Source: CAD feature listing. Evaluate the final solid. Frame: model axes, mm. A direction names the side the tool comes from. Coordinates: 2 decimals unless noted, no trailing zeros. Loops run counter-clockwise (first coordinate to the right, second up) from the corner with the lowest first, then second, coordinate; pieces in that order, holes last. Notation, with made-up numbers: (36.25, -22.5) -> (80.25, -22.5) arc R8 cw to (80.25, -11.5) -> close; hole circle Ø7 at (82.5, -18). An arc over 180 degrees is marked (long way). Answer as a JSON object with one key per item and string values. Group by question number.
from build123d import *

# Parameters (mm, degrees)
F0_W     = 450
F0_H     = 450
F1_DEPTH = 950
F2_W     = 50
F2_H     = 50
F2_H_2   = 425
F2_W_2   = 330
F3_DEPTH = 450.001
F4_W     = 380
F4_H     = 425
F5_DEPTH = 450.001
F6_W     = 380
F6_H     = 50
F6_H_2   = 306.2882968217
F7_DEPTH = 134.2592361444


with BuildPart() as f1:
    # F0 (on Top) → F1 (new body)
    with BuildSketch(Plane.XY):
        Rectangle(F0_W, F0_H)
    extrude(amount=F1_DEPTH)

    # F2 (on face) → F3 (cut, through all)
    with BuildSketch(Plane.YZ.offset(225)):
        Polygon((-225, 475), (140, 475), (190, 950), (-225, 950), align=None)
        Polygon((175, 475), (225, 475), (225, 950), align=None)
        with Locations((200, 450)):
            Rectangle(F2_W, F2_H)
        with Locations((200, 212.5)):
            Rectangle(F2_W, F2_H_2)
        with Locations((-25, 212.5)):
            Rectangle(F2_W_2, F2_H_2)
    extrude(amount=-F3_DEPTH, mode=Mode.SUBTRACT)

    # F4 (on face) → F5 (cut, through all)
    with BuildSketch(Plane.XZ.offset(225)):
        with Locations((0, 212.5)):
            Rectangle(F4_W, F4_H)
    extrude(amount=-F5_DEPTH, mode=Mode.SUBTRACT)

    # F6 (on face) → F7 (cut, through all)
    with BuildSketch(Plane(origin=(0, 89.0136986301, -9.3698630137), x_dir=(1, 0, 0), z_dir=(0, -0.9945054529, 0.1046847845))):
        with Locations((0, 868.3342567919)):
            Rectangle(F6_W, F6_H)
        with Locations((0, 640.190108381)):
            Rectangle(F6_W, F6_H_2)
    extrude(amount=-F7_DEPTH, mode=Mode.SUBTRACT)


solid = f1.part
1. Section query B-B on x = 179. Return loops of the section in (y, z).
2. Section query A-A on z = 402.5. Return loops of the section in (x, y), then the cut area to 3 significant figures.
3. Reachability of faces 4 (the face through (-190, -208, 210)), 5 (the face through (207, -207, 0)), 6 (the face through (-3, 208, 950)), 7 (the face through (-207, -190, 210)), 8 (the face through (1, 175, 432)) from +Z, -Z, +X, -X, +Y, -Y: full face, straight path, thin tool, end or side. Return the list, or none.
4. Ray query, L1, parallel to Z at x = -122.5, y = -173.5; L2, parallel to Z at x = -105.5, y = 204; L3, parallel to Y at x = 135, z = 452.5. Return the intervals inside material, ascending.
5. Mould query, pull axis Z, two halves, no side actions, for faces 1 (the face through (208, 140, 210)), 2 (the face through (3, -45, 475)), 3 (the face through (-2.66, 199.6, 877.26)). Classes: pulls with the +Z half, pulls with the -Z half, needs draft (parallel to the pull), parting line crosses it, or undercut.
6. Section query D-D on y = -155.5. Return loops of the section in (x, z).
7. Section query C-C on z = 709. Return loops of the section in (x, y), then the cut area to 3 significant figures.
8. Pin query (flat end, axial travel): pin 1 Ø4 at (x, y) = (143, -75.5) entering from -Z; pin 2 Ø6 at (x, y) = (-27, -2) entering from +Z; pin 3 Ø10.5 at (x, z) = (211, 187) entering from +Y. Return the tip coordinate at first contact, or that it passes through.
Solved:
{
 "1": {"outline": "(-225, 425) -> (175, 425) -> (175, 471.32) -> (140, 475) -> (-225, 475) -> close; (172.06, 779.61) -> (206.68, 775.96) -> (211.91, 825.69) -> (177.3, 829.33) -> close; (182.53, 879.06) -> (217.15, 875.41) -> (225, 950) -> (190, 950) -> close"},
 "2": {"outline": "(-225, -225) -> (-190, -225) -> (-190, -190) -> (-225, -190) -> close; (-225, 140) -> (-190, 140) -> (-190, 175) -> (-225, 175) -> close; (190, -225) -> (225, -225) -> (225, -190) -> (190, -190) -> close; (190, 140) -> (225, 140) -> (225, 175) -> (190, 175) -> close", "area": "4,900 mm^2"},
 "3": {"face 4": "-Z, +Y, -Y", "face 5": "-Z, +X, -X, +Y, -Y", "face 6": "+Z, +X, -X, +Y, -Y", "face 7": "-Z, +X, -X", "face 8": "-Z, +X, -X, +Y"},
 "4": {"L1": "425 to 475", "L2": "776.24 to 826.52, 876.8 to 950", "L3": "-225 to 175"},
 "5": {"face 1": "needs draft", "face 2": "pulls with the +Z half", "face 3": "undercut"},
 "6": {"outline": "(-225, 425) -> (225, 425) -> (225, 475) -> (-225, 475) -> close"},
 "7": {"outline": "(-225, 164.63) -> (-190, 164.63) -> (-190, 199.63) -> (-225, 199.63) -> close; (190, 164.63) -> (225, 164.63) -> (225, 199.63) -> (190, 199.63) -> close", "area": "2,450 mm^2"},
 "8": {"pin 1": "z = 425", "pin 2": "z = 475", "pin 3": "y = 175"}
}
